CAD build for the part. Positions are in the model's coordinates, mm. Face numbers are marked on the shaded views. A direction names the side the tool comes from. Give positions to 0.01 mm unless a question says otherwise; leave off trailing zeros. Write each loop counter-clockwise with the first axis right and the second up, starting at its lowest first coordinate (ties: lowest second). Pieces come first, ordered by that corner, then holes. Notation, with made-up numbers: (-7, 60.25) -> (42, 60.25) arc R22 ccw to (42, 86.25) -> close; hole circle Ø3 at (45.5, 39). An arc over 180 degrees is marked (long way). Answer as a JSON object with one key per item and string values.
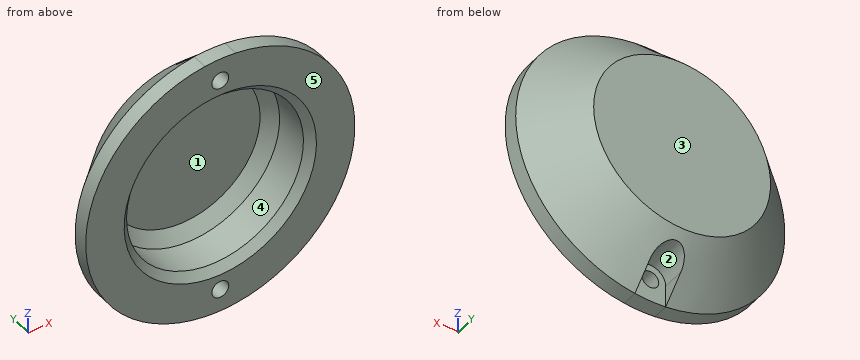
```python
from build123d import *
from build123d.topology import SkipClean

# Parameters (mm, degrees)
BOSS_EXTRUDE1_DEPTH = 2
SKETCH2_R           = 11.5
BOSS_EXTRUDE2_DEPTH = 6
CHAMFER1_START      = 2
CHAMFER1_2_DEPTH    = 6
SKETCH6_R           = 17.5
SKETCH6_R_2         = 1.1
BOSS_EXTRUDE3_DEPTH = 2
SKETCH7_R           = 11.5
CUT_EXTRUDE1_DEPTH  = 7
CHAMFER2_SIZE       = 1.5
CHAMFER3_SIZE       = 1


with BuildPart() as part:
    # Sketch1 → Boss-Extrude1 (new body)
    with BuildSketch(Plane(origin=(0, 0, 0), x_dir=(1, 0, 0), z_dir=(0, 1, 0))):
        with BuildLine():
            Line((-2, 14.5), (-2, 17.385338651))
            ThreePointArc((-2, 17.385338651), (-17.5, 0), (-2, -17.385338651))
            Line((-2, -17.385338651), (-2, -14.5))
            ThreePointArc((-2, -14.5), (0, -12.5), (2, -14.5))
            Line((2, -14.5), (2, -17.385338651))
            ThreePointArc((2, -17.385338651), (17.5, 0), (2, 17.385338651))
            Line((2, 17.385338651), (2, 14.5))
            ThreePointArc((2, 14.5), (0, 12.5), (-2, 14.5))
        make_face()
    extrude(amount=BOSS_EXTRUDE1_DEPTH)

    # Sketch2 → Boss-Extrude2 (add)
    with BuildSketch(Plane(origin=(0, 2, 0), x_dir=(1, 0, 0), z_dir=(0, 1, 0))):
        with Locations(Location((0, 0, 0), (0, 0, 270))):
            Circle(SKETCH2_R)
    extrude(amount=BOSS_EXTRUDE2_DEPTH)

    # Chamfer1: read off the stored shape, not the designer's step
    # Chamfer1 outline → Chamfer1 (revolve)
    with BuildSketch(Plane.XY):
        Polygon((17.5, 2), (11.5, 8), (11.5, 2), align=None)
    revolve(axis=Axis((0, 0, 0), (0, 1, 0)))

    # Chamfer1 2 outline → Chamfer1 2 (cut)
    with BuildSketch(Plane(origin=(0, 0, 0), x_dir=(1, 0, 0), z_dir=(0, 1, 0)).offset(CHAMFER1_START)):
        with BuildLine():
            ThreePointArc((2, -14.5), (0, -12.5), (-2, -14.5))
            Line((-2, -14.5), (-2, -19))
            Line((-2, -19), (2, -19))
            Line((2, -19), (2, -14.5))
        make_face()
        with BuildLine():
            Line((2, 19), (-2, 19))
            Line((-2, 19), (-2, 14.5))
            ThreePointArc((-2, 14.5), (0, 12.5), (2, 14.5))
            Line((2, 14.5), (2, 19))
        make_face()
    extrude(amount=CHAMFER1_2_DEPTH, mode=Mode.SUBTRACT)

    # Sketch6 → Boss-Extrude3 (add)
    with SkipClean():  # the faces are left unmerged after this step: merging them gives an invalid solid
        with BuildSketch(Plane.XZ):
            with Locations(Location((0, 0, 0), (0, 0, 263.437572131))):
                Circle(SKETCH6_R)
            with Locations(Location((0, 14.5, 0), (0, 0, 270))):
                Circle(SKETCH6_R_2, mode=Mode.SUBTRACT)
            with Locations(Location((0, -14.5, 0), (0, 0, 270))):
                Circle(SKETCH6_R_2, mode=Mode.SUBTRACT)
        extrude(amount=-BOSS_EXTRUDE3_DEPTH)

    # Sketch7 → Cut-Extrude1 (cut)
    with SkipClean():  # the faces are left unmerged after this step: merging them gives an invalid solid
        with BuildSketch(Plane.XZ):
            with Locations(Location((0, 0, 0), (0, 0, 270))):
                Circle(SKETCH7_R)
        extrude(amount=-CUT_EXTRUDE1_DEPTH, mode=Mode.SUBTRACT)

    # Chamfer2
    chamfer2_edges = [part.edges().sort_by_distance(p)[0] for p in [
        (0, 7, 11.5),
    ]]
    chamfer(chamfer2_edges, length=CHAMFER2_SIZE)

    # Chamfer3
    chamfer3_edges = [part.edges().sort_by_distance(p)[0] for p in [
        (0, 0, 11.5),
    ]]
    chamfer(chamfer3_edges, length=CHAMFER3_SIZE - 0.0001)  # a hair under: the kernel refuses the full size


solid = part.part
```
1) Mould opens along Z. For the marked faces 1, 2 and 3 say: released by +Z, released by -Z, zero draft, split by the parting line, or undercut.
Model answer:
{"face 1": "undercut", "face 2": "released by -Z", "face 3": "zero draft"}
2) 3-axis set-ups, long thin cutter, end or side, ignore diameter. For the marked faces 4 and 5: which of +Z, -Z, +X, -X, +Y, -Y reach the whole face in a straight line?
Model answer:
{"face 4": "-Y", "face 5": "+Z, -Z, +X, -X, -Y"}
3) Slice it at A-A (x = 0). List the corners of the cut face in (y, z).
Model answer:
{"outline": "(0, -17.5) -> (2, -17.5) -> (2, -15.6) -> (0, -15.6) -> close; (0, -13.4) -> (2, -13.4) -> (2, -12.5) -> (7, -12.5) -> (8, -11.5) -> (8, 11.5) -> (7, 12.5) -> (2, 12.5) -> (2, 13.4) -> (0, 13.4) -> (0, 12.5) -> (1, 11.5) -> (5.5, 11.5) -> (7, 10) -> (7, -10) -> (5.5, -11.5) -> (1, -11.5) -> (0, -12.5) -> close; (0, 15.6) -> (2, 15.6) -> (2, 17.5) -> (0, 17.5) -> close"}
4) Pin check, flat tips, straight feed: pin 1 (1.2 mm diameter, centred on x = 0.5, z = -16, fed in from +Y); pin 2 (3 mm diameter, centred on y = 3, z = -16, fed in from -X); pin 3 (1.5 mm diameter, centred on x = -5.5, y = 4, fed in from +Z). Stop position of each tip, or through.
Model answer:
{"pin 1": "stops at y = 2", "pin 2": "stops at x = -9.21", "pin 3": "stops at z = 15.33"}
5) Slice it at B-B (y = 7.5). List the corners of the cut face in (x, z), then the cut area to 3 significant figures.
Model answer:
{"outline": "circle Ø24 at (0, 0)", "area": "452 mm2"}
6) Wall check: probe 1 along Z at (x, y) = (-9.5, 6.25); probe 2 along Y at (x, z) = (8, -1); probe 3 along X at (y, z) = (0.5, 15). Give the ranges that are in metal, low to high.
Model answer:
{"probe 1": "z = -9.24 to -5.03, 5.03 to 9.24", "probe 2": "y = 7 to 8", "probe 3": "x = -9.01 to -0.98, 0.98 to 9.01"}
